The listing builds one solid part. Answer for the finished solid, in the listing's coordinates (mm). Face numbers are marked on the shaded views. A direction names the side the tool comes from. Give positions to 0.01 mm unless a question says otherwise; leave off trailing zeros. Write each loop counter-clockwise with the first axis right and the second up, starting at its lowest first coordinate (ties: lowest second). Pieces come first, ordered by that corner, then holes.
```python
from build123d import *

# Parameters (mm, degrees)
F1_DEPTH       = 25.4
F2_DEPTH       = 25.4
F4_D           = 25.4
F4_CBORE_D     = 38.1
F4_CBORE_DEPTH = 12.7
F5_DEPTH       = 25.4
F6_DEPTH       = 25.4
F8_D           = 30.48
F8_CBORE_D     = 43.18
F8_CBORE_DEPTH = 43.18


with BuildPart() as f1:
    # F0 (on Front) → F1 (new body)
    with BuildSketch(Plane.XZ):
        with BuildLine():
            ThreePointArc((-6.0617997533, 50.4444008589), (-47.1386495735, 91.5212506791), (-88.2154993937, 50.4444008589))
            Line((-88.2154993937, 50.4444008589), (-68.9775327914, 50.4444008589))
            ThreePointArc((-68.9775327914, 50.4444008589), (-47.1386495735, 72.2832840767), (-25.2997663556, 50.4444008589))
            Line((-25.2997663556, 50.4444008589), (-6.0617997533, 50.4444008589))
        make_face()
        with BuildLine():
            Line((-68.9775327914, 50.4444008589), (-88.2154993937, 50.4444008589))
            ThreePointArc((-88.2154993937, 50.4444008589), (-47.1386495735, 9.3675510387), (-6.0617997533, 50.4444008589))
            Line((-6.0617997533, 50.4444008589), (-25.2997663556, 50.4444008589))
            ThreePointArc((-25.2997663556, 50.4444008589), (-47.1386495735, 28.605517641), (-68.9775327914, 50.4444008589))
        make_face()
        with BuildLine():
            Line((-88.2866495735, 50.4444008589), (-88.2866495735, -25.7555991411))
            Line((-88.2866495735, -25.7555991411), (89.5133504265, -25.7555991411))
            Line((89.5133504265, -25.7555991411), (89.5133504265, 2.6924008589))
            Line((89.5133504265, 2.6924008589), (-5.9906495735, 2.6924008589))
            Line((-5.9906495735, 2.6924008589), (-5.9906495735, 50.4444008589))
            Line((-5.9906495735, 50.4444008589), (-6.0617997533, 50.4444008589))
            ThreePointArc((-6.0617997533, 50.4444008589), (-47.1386495735, 9.3675510387), (-88.2154993937, 50.4444008589))
            Line((-88.2154993937, 50.4444008589), (-88.2866495735, 50.4444008589))
        make_face()
    extrude(amount=F1_DEPTH)

    # F2 (add): a face of the model
    f2_faces = [f1.faces().sort_by_distance(p)[0] for p in [
        (-23.3187363133, -25.4, 14.8327425436),
    ]]
    extrude(f2_faces, amount=F2_DEPTH)

    # F4 (through all)
    with Locations(Plane.XY.offset(2.6924008589)):
        with Locations((41.4565503597, -24.5364010334)):
            CounterBoreHole(F4_D / 2, F4_CBORE_D / 2, F4_CBORE_DEPTH)

    # F0 (on Front) → F5 (join)
    with BuildSketch(Plane.XZ):
        with BuildLine():
            Line((-47.1386495735, 50.4444008589), (-68.9775327914, 50.4444008589))
            ThreePointArc((-68.9775327914, 50.4444008589), (-47.1386495735, 28.605517641), (-25.2997663556, 50.4444008589))
            Line((-25.2997663556, 50.4444008589), (-47.1386495735, 50.4444008589))
        make_face()
        with BuildLine():
            ThreePointArc((-25.2997663556, 50.4444008589), (-47.1386495735, 72.2832840767), (-68.9775327914, 50.4444008589))
            Line((-68.9775327914, 50.4444008589), (-47.1386495735, 50.4444008589))
            Line((-47.1386495735, 50.4444008589), (-25.2997663556, 50.4444008589))
        make_face()
    extrude(amount=F5_DEPTH)

    # F6 (add): a face of the model
    f6_faces = [f1.faces().sort_by_distance(p)[0] for p in [
        (-47.1386495735, -25.4, 50.4444008589),
    ]]
    extrude(f6_faces, amount=F6_DEPTH)

    # F8 (through all)
    with Locations(Plane.XZ.offset(50.8)):
        with Locations((-47.1386495735, 50.4444008589)):
            CounterBoreHole(F8_D / 2, F8_CBORE_D / 2, F8_CBORE_DEPTH)


solid = f1.part
```
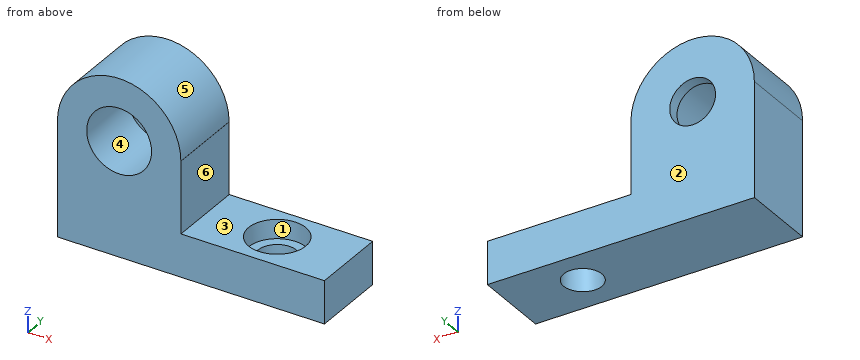
Item 1: Determine the mould class of the marked faces 4, 5 and 6 for opening direction Z: pulls with the +Z half, pulls with the -Z half, needs draft (parallel to the pull), parting line crosses it, or undercut.
Conclusion:
face 4: undercut
face 5: pulls with the +Z half
face 6: needs draft
Item 2: Which of the six approach directions +Z, -Z, +X, -X, +Y, -Y give full straight-line access (tool end or side, diameter ignored) to the marked faces 1, 2 and 3?
Conclusion:
face 1: +Z
face 2: +Z, -Z, +X, -X, +Y
face 3: +Z, +X, +Y, -Y
Item 3: Consider probe 1 along Z at (x, y) = (-46.5, -48); probe 2 along Z at (x, y) = (77.5, -7); probe 3 along Y at (x, z) = (-37, 32.5). Determine where each line is inside the solid, lowest interval first.
Conclusion:
probe 1: z = -25.76 to 28.86, 72.02 to 91.52
probe 2: z = -25.76 to 2.69
probe 3: y = -7.62 to 0
Item 4: A cutting plane is placed at B-B, the plane z = 56.5. Give the vertices of the cut face in (x, y), plus the area to 4 significant figures.
Conclusion:
outline: (-87.77, -50.8) - (-67.86, -50.8) - (-67.86, -7.62) - (-61.12, -7.62) - (-61.12, 0) - (-87.77, 0) - close; (-33.15, -7.62) - (-26.42, -7.62) - (-26.42, -50.8) - (-6.51, -50.8) - (-6.51, 0) - (-33.15, 0) - close
area: 2,125 mm2
Item 5: A cutting plane is placed at C-C, the plane x = -41.5. Give the vertices of the cut face in (y, z), plus the area to 3 significant figures.
Conclusion:
outline: (-50.8, -25.76) - (0, -25.76) - (0, 36.29) - (-7.62, 36.29) - (-7.62, 29.6) - (-50.8, 29.6) - close; (-50.8, 71.29) - (-7.62, 71.29) - (-7.62, 64.6) - (0, 64.6) - (0, 91.13) - (-50.8, 91.13) - close
area: 3,920 mm2
Item 6: Each of these flat-tipped pins is pushed along its axis until it touches: P1, Ø11.5, axis at x = 47.5, y = -18, coming from the +Z side; P2, Ø14.5, axis at y = -22, z = 21, coming from the +X side; P3, Ø12, axis at x = 62.5, y = -19.5, coming from the +Z side. Where does it stop, or does it pass through?
Conclusion:
P1: stops at z = -10.01
P2: stops at x = -5.99
P3: stops at z = 2.69
Item 7: A cutting plane is placed at A-A, the plane y = -22. Give the vertices of the cut face in (x, z), plus the area to 3 significant figures.
Conclusion:
outline: (-88.29, -25.76) - (29.01, -25.76) - (29.01, -10.01) - (22.58, -10.01) - (22.58, 2.69) - (-5.99, 2.69) - (-5.99, 50.44) - (-6.06, 50.44) arc R41.08 ccw to (-88.22, 50.44) - (-88.29, 50.44) - close; (53.9, -25.76) - (89.51, -25.76) - (89.51, 2.69) - (60.34, 2.69) - (60.34, -10.01) - (53.9, -10.01) - close; hole circle Ø43.18 at (-47.14, 50.44)
area: 9,300 mm2
Item 8: A cutting plane is placed at D-D, the plane y = -35. Give the vertices of the cut face in (x, z).
Conclusion:
outline: (-88.29, -25.76) - (34.26, -25.76) - (34.26, -10.01) - (25.54, -10.01) - (25.54, 2.69) - (-5.99, 2.69) - (-5.99, 50.44) - (-6.06, 50.44) arc R41.08 ccw to (-88.22, 50.44) - (-88.29, 50.44) - close; (48.65, -25.76) - (89.51, -25.76) - (89.51, 2.69) - (57.38, 2.69) - (57.38, -10.01) - (48.65, -10.01) - close; hole circle Ø43.18 at (-47.14, 50.44)
